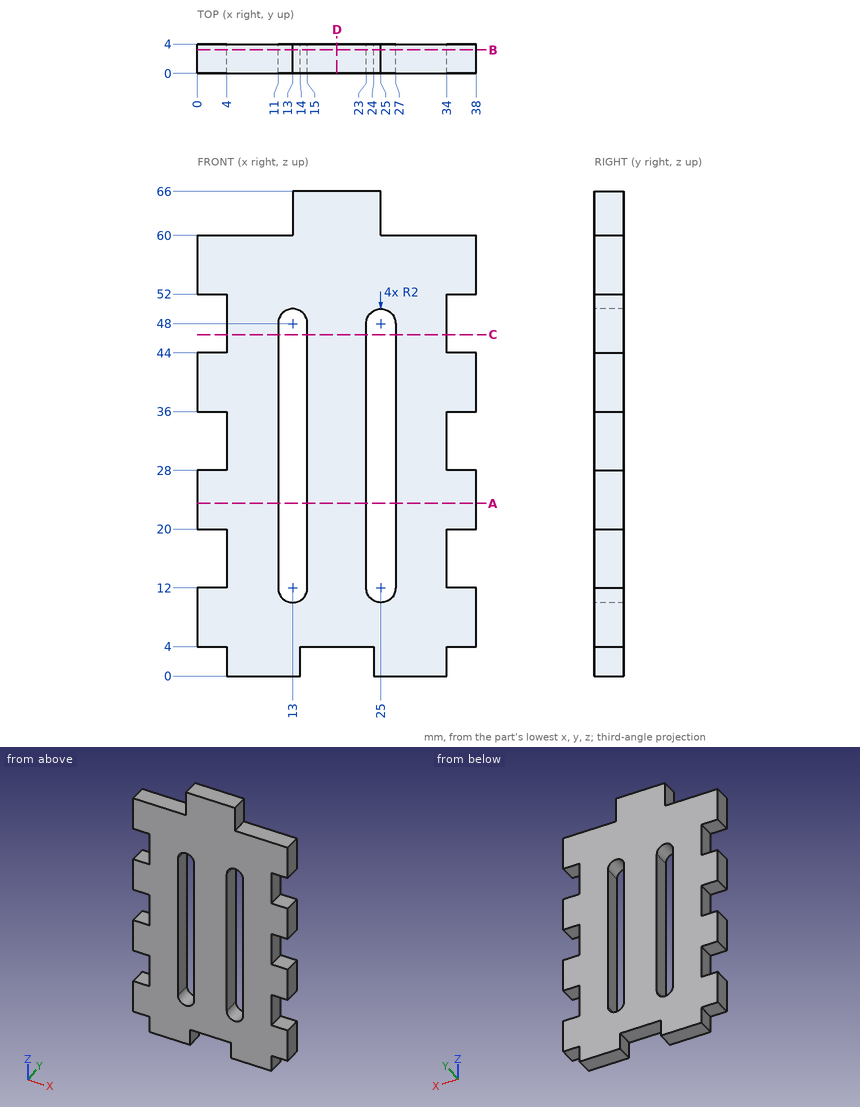
Print and shaded views of the part. All mm, measured from the part's lowest x, y and z. Coordinates: 2 decimals unless noted, no trailing zeros. Loops run counter-clockwise (first coordinate to the right, second up) from the corner with the lowest first, then second, coordinate; pieces in that order, holes last. Notation, with made-up numbers: (-31, -38) - (14, -38) arc R13 cw to (14, -31) - close; hole circle Ø10 at (65.25, -21.75). An arc over 180 degrees is marked (long way). Write item = value, one per line. Start each with the question number.
Item 1: Saw through at A-A, the plane z = 23.5. List the corners of the cut face in (x, y).
Item 2: Saw through at B-B, the plane y = 3.2. State how many separate pieces and enclosed holes the cut face has, then the cut area to 3 significant figures.
Item 3: Drop flat-ended pins along their axis: pin 1 Ø2 at (x, y) = (2.5, 2.5) entering from -Z; pin 2 Ø2 at (y, z) = (2, 30) entering from +X; pin 3 Ø1.2 at (y, z) = (2, 15.5) entering from -X. Give the stop position or say it passes through.
Item 4: Saw through at D-D, the plane x = 19. List the corners of the cut face in (y, z).
Item 5: Wall check: probe 1 along X at (y, z) = (1.15, 42.5); probe 2 along X at (y, z) = (2.15, 16); probe 3 along X at (y, z) = (2.1, 50.5). Give the ranges that are in metal, low to high. Write a range as [from, to].
Item 6: Saw through at C-C, the plane z = 46.5. List the corners of the cut face in (x, y).
Answers:
q1.outline = (0, 0) - (11, 0) - (11, 4) - (0, 4) - close; (15, 0) - (23, 0) - (23, 4) - (15, 4) - close; (27, 0) - (38, 0) - (38, 4) - (27, 4) - close
q2.separate_pieces = 1
q2.enclosed_holes = 2
q2.area = 1,770 mm2
q3.pin_1 = 4
q3.pin_2 = 34
q3.pin_3 = 4
q4.outline = (0, 4) - (4, 4) - (4, 66) - (0, 66) - close
q5.probe_1 = [0, 11], [15, 23], [27, 38]
q5.probe_2 = [4, 11], [15, 23], [27, 34]
q5.probe_3 = [4, 34]
q6.outline = (4, 0) - (11, 0) - (11, 4) - (4, 4) - close; (15, 0) - (23, 0) - (23, 4) - (15, 4) - close; (27, 0) - (34, 0) - (34, 4) - (27, 4) - close
